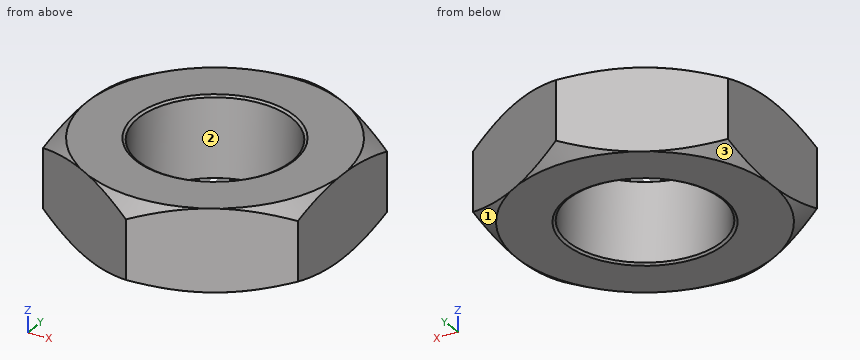
```python
from build123d import *

# Parameters (mm, degrees)
SKETCH3_R                    = 3
BOSS_EXTRUDE1_DEPTH          = 1.6
SKETCH4_OUTSIDE_W            = 49.762
SKETCH4_OUTSIDE_H            = 51.31
SKETCH4_OUTSIDE_R            = 5
CUT_EXTRUDE1_DEPTH           = 10
CUT_EXTRUDE1_DRAFT           = -60
SKETCH4_OUTSIDE_R_2          = 3.108253175
CUT_EXTRUDE1_PROFILE_2_DEPTH = 10
CUT_EXTRUDE1_PROFILE_2_DRAFT = -60
MIRROR1_COPY_1_SKETCH_W      = 49.762
MIRROR1_COPY_1_SKETCH_H      = 51.31
MIRROR1_COPY_1_SKETCH_R      = 5
MIRROR1_COPY_1_DEPTH         = 10
MIRROR1_COPY_1_DRAFT         = -60
MIRROR1_COPY_2_SKETCH_R      = 3.108253175
MIRROR1_COPY_2_DEPTH         = 10
MIRROR1_COPY_2_DRAFT         = -60
MIRROR1_COPY_3_SKETCH_R      = 3.108253175
MIRROR1_COPY_3_DEPTH         = 10
MIRROR1_COPY_3_DRAFT         = -60


with BuildPart() as part:
    # Sketch3 → Boss-Extrude1 (new, symmetric)
    with BuildSketch(Plane.XY):
        Polygon((-5, 2.886751346), (-5, -2.886751346), (0, -5.773502692), (5, -2.886751346), (5, 2.886751346), (0, 5.773502692), align=None)
        Circle(SKETCH3_R, mode=Mode.SUBTRACT)
    extrude(amount=BOSS_EXTRUDE1_DEPTH, both=True)


with BuildPart() as cut_extrude1_tool:
    # Sketch4 outside → Cut-Extrude1 (with draft: the straight prism first)
    with BuildSketch(Plane.XY.offset(1.6)):
        Rectangle(SKETCH4_OUTSIDE_W, SKETCH4_OUTSIDE_H)
        Circle(SKETCH4_OUTSIDE_R, mode=Mode.SUBTRACT)
    extrude(amount=-CUT_EXTRUDE1_DEPTH)
    # Cut-Extrude1: the draft: its side faces are tilted about the plane it starts from
    cut_extrude1_sides = [cut_extrude1_tool.faces().sort_by_distance(p)[0] for p in [
        (0, -25.655, -3.4),
        (24.881, 0, -3.4),
        (0, 25.655, -3.4),
        (-24.881, 0, -3.4),
        (-5, 0, -3.4),
    ]]
    draft(cut_extrude1_sides, Plane.XY.offset(1.6), CUT_EXTRUDE1_DRAFT)


with BuildPart() as part_1:
    add(part.part)

    # Cut-Extrude1: cut by cut_extrude1_tool
    add(cut_extrude1_tool.part, mode=Mode.SUBTRACT)


with BuildPart() as cut_extrude1_profile_2_tool:
    # Sketch4 outside → Cut-Extrude1 profile 2 (with draft: the straight prism first)
    with BuildSketch(Plane.XY.offset(1.6)):
        Circle(SKETCH4_OUTSIDE_R_2)
    extrude(amount=-CUT_EXTRUDE1_PROFILE_2_DEPTH)
    # Cut-Extrude1 profile 2: the draft: its side faces are tilted about the plane it starts from
    cut_extrude1_profile_2_sides = [cut_extrude1_profile_2_tool.faces().sort_by_distance(p)[0] for p in [
        (-3.108253175, 0, -3.4),
    ]]
    draft(cut_extrude1_profile_2_sides, Plane.XY.offset(1.6), CUT_EXTRUDE1_PROFILE_2_DRAFT)


with BuildPart() as part_2:
    add(part_1.part)

    # Cut-Extrude1 profile 2: cut by cut_extrude1_profile_2_tool
    add(cut_extrude1_profile_2_tool.part, mode=Mode.SUBTRACT)


with BuildPart() as mirror1_copy_1_tool:
    # Mirror1 copy 1 sketch → Mirror1 copy 1 (with draft: the straight prism first)
    with BuildSketch(Plane(origin=(0, 0, -1.6), x_dir=(1, 0, 0), z_dir=(0, 0, -1))):
        Rectangle(MIRROR1_COPY_1_SKETCH_W, MIRROR1_COPY_1_SKETCH_H)
        Circle(MIRROR1_COPY_1_SKETCH_R, mode=Mode.SUBTRACT)
    extrude(amount=-MIRROR1_COPY_1_DEPTH)
    # Mirror1 copy 1: the draft: its side faces are tilted about the plane it starts from
    mirror1_copy_1_sides = [mirror1_copy_1_tool.faces().sort_by_distance(p)[0] for p in [
        (0, -25.655, 3.4),
        (24.881, 0, 3.4),
        (0, 25.655, 3.4),
        (-24.881, 0, 3.4),
        (-5, 0, 3.4),
    ]]
    draft(mirror1_copy_1_sides, Plane(origin=(0, 0, -1.6), x_dir=(1, 0, 0), z_dir=(0, 0, -1)), MIRROR1_COPY_1_DRAFT)


with BuildPart() as part_3:
    add(part_2.part)

    # Mirror1 copy 1: cut by mirror1_copy_1_tool
    add(mirror1_copy_1_tool.part, mode=Mode.SUBTRACT)


with BuildPart() as mirror1_copy_2_tool:
    # Mirror1 copy 2 sketch → Mirror1 copy 2 (with draft: the straight prism first)
    with BuildSketch(Plane(origin=(0, 0, -1.6), x_dir=(1, 0, 0), z_dir=(0, 0, -1))):
        Circle(MIRROR1_COPY_2_SKETCH_R)
    extrude(amount=-MIRROR1_COPY_2_DEPTH)
    # Mirror1 copy 2: the draft: its side faces are tilted about the plane it starts from
    mirror1_copy_2_sides = [mirror1_copy_2_tool.faces().sort_by_distance(p)[0] for p in [
        (-3.108253175, 0, 3.4),
    ]]
    draft(mirror1_copy_2_sides, Plane(origin=(0, 0, -1.6), x_dir=(1, 0, 0), z_dir=(0, 0, -1)), MIRROR1_COPY_2_DRAFT)


with BuildPart() as part_4:
    add(part_3.part)

    # Mirror1 copy 2: cut by mirror1_copy_2_tool
    add(mirror1_copy_2_tool.part, mode=Mode.SUBTRACT)


with BuildPart() as mirror1_copy_3_tool:
    # Mirror1 copy 3 sketch → Mirror1 copy 3 (with draft: the straight prism first)
    with BuildSketch(Plane(origin=(0, 0, -1.6), x_dir=(1, 0, 0), z_dir=(0, 0, -1))):
        Circle(MIRROR1_COPY_3_SKETCH_R)
    extrude(amount=-MIRROR1_COPY_3_DEPTH)
    # Mirror1 copy 3: the draft: its side faces are tilted about the plane it starts from
    mirror1_copy_3_sides = [mirror1_copy_3_tool.faces().sort_by_distance(p)[0] for p in [
        (-3.108253175, 0, 3.4),
    ]]
    draft(mirror1_copy_3_sides, Plane(origin=(0, 0, -1.6), x_dir=(1, 0, 0), z_dir=(0, 0, -1)), MIRROR1_COPY_3_DRAFT)


with BuildPart() as part_5:
    add(part_4.part)

    # Mirror1 copy 3: cut by mirror1_copy_3_tool
    add(mirror1_copy_3_tool.part, mode=Mode.SUBTRACT)


solid = part_5.part
```
Check sheet for the modelled part. Datum: model origin and axes. Units: mm. Face numbers are marked on the shaded views. Give positions to 0.01 mm unless a question says otherwise; leave off trailing zeros. Loops run counter-clockwise (first coordinate to the right, second up) from the corner with the lowest first, then second, coordinate; pieces in that order, holes last. Notation, with made-up numbers: M 3,58 L 28,58 A10 cw 28,62 Z; hole C 61.5,-34.75 d3. An arc over 180 degrees is marked long. Answer in a Markdown table with one row per item.
1) Mould release check, pull along X, two halves, no side actions. Record for the marked faces 1, 2 and 3: released by +X, released by -X, zero draft, split by the parting line, or undercut.
Solutions:
| item | result |
|---|---|
| face 1 | released by +X |
| face 2 | undercut |
| face 3 | released by -X |
2) Depth check by flat-ended pin: pin 1 (5.5 mm diameter, centred on x = 0, y = 0, fed in from -Z); pin 2 (1.5 mm diameter, centred on x = 2, z = -1, fed in from +Y). Enter the tip coordinate at first touch or a pass-through.
Solutions:
| item | result |
|---|---|
| pin 1 | passes through |
| pin 2 | stops at y = 5.05 |
3) Cross-section at A-A (z = -0.95). Enter the section's corners in (x, y).
Solutions:
| item | result |
|---|---|
| outline | M -5,-2.89 L 0,-5.77 L 5,-2.89 L 5,2.89 L 0,5.77 L -5,2.89 Z; hole C 0,0 d6 |
4) Thickness scan on line 1 (X direction, y = 0, z = 0.4); line 2 (X direction, y = 2, z = 0.95); line 3 (Y direction, x = 2.25, z = 1.45). Record the ranges inside material, lowest first.
Solutions:
| item | result |
|---|---|
| line 1 | x = -5 to -3, 3 to 5 |
| line 2 | x = -5 to -2.24, 2.24 to 5 |
| line 3 | y = -4.47 to -1.98, 1.98 to 4.47 |
